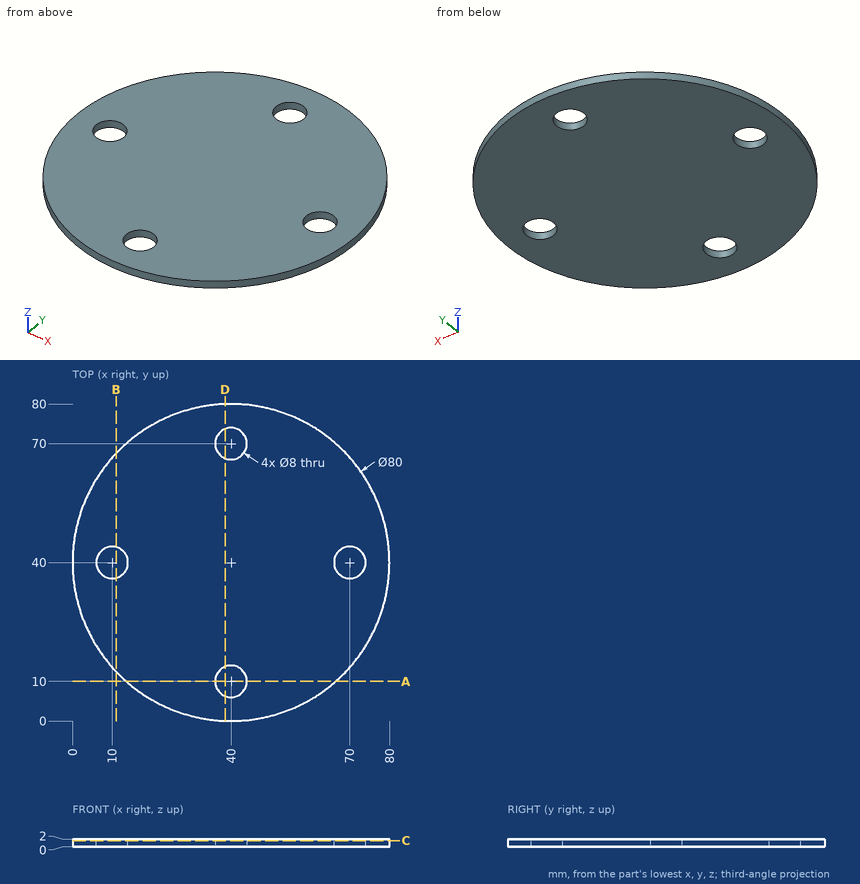
Could you check a few things on this drawing? It's one solid part, dimensions in mm from its lowest x, y, z. Coordinates: 2 decimals unless noted, no trailing zeros. Loops run counter-clockwise (first coordinate to the right, second up) from the corner with the lowest first, then second, coordinate; pieces in that order, holes last. Notation, with made-up numbers: (-35.5, 59) - (21.5, 59) arc R13 cw to (21.5, 83) - close; hole circle Ø8 at (41.5, 76.5). An arc over 180 degrees is marked (long way). Return JSON: item names as keys, results as strings. Group by question number.
Item 1: I need wall thicknesses on line 1 (Y direction, x = 40, z = 1.65); line 2 (X direction, y = 12.5, z = 1.05); line 3 (Y direction, x = 72, z = 1.85). Which ranges of each line are inside material? Lowest first, please. Write a range as from..to.
Item 2: If we section it at B-B on x = 11: Write out the boundary of the cut face in (y, z), and give its area (3 significant figures).
Item 3: Will this pin go through, and if not, where does the flat tip stop? P1, Ø1, axis at x = 49, z = 1.5, coming from the -Y side.
Item 4: If we section it at D-D on x = 38.5: Write out the boundary of the cut face in (y, z), and give its area (3 significant figures).
Item 5: If we section it at C-C on z = 1.6: Write out the boundary of the cut face in (x, y), and give its area (3 significant figures).
Item 6: If we section it at A-A on y = 10: Write out the boundary of the cut face in (x, z).
Calculated:
{
 "1": {"line 1": "y = 0..6, 14..66, 74..80", "line 2": "x = 10.95..36.88, 43.12..69.05", "line 3": "y = 16..36.54, 43.46..64"},
 "2": {"outline": "(12.45, 0) - (36.13, 0) - (36.13, 2) - (12.45, 2) - close; (43.87, 0) - (67.55, 0) - (67.55, 2) - (43.87, 2) - close", "area": "94.7 mm^2"},
 "3": {"P1": "stops at y = 0.91"},
 "4": {"outline": "(0.03, 0) - (6.29, 0) - (6.29, 2) - (0.03, 2) - close; (13.71, 0) - (66.29, 0) - (66.29, 2) - (13.71, 2) - close; (73.71, 0) - (79.97, 0) - (79.97, 2) - (73.71, 2) - close", "area": "130 mm^2"},
 "5": {"outline": "circle Ø80 at (40, 40); hole circle Ø8 at (10, 40); hole circle Ø8 at (40, 10); hole circle Ø8 at (40, 70); hole circle Ø8 at (70, 40)", "area": "4,830 mm^2"},
 "6": {"outline": "(13.54, 0) - (36, 0) - (36, 2) - (13.54, 2) - close; (44, 0) - (66.46, 0) - (66.46, 2) - (44, 2) - close"}
}
